CAD build for the part. Positions are in the model's coordinates, mm. Face numbers are marked on the shaded views. Round coordinates to 2 decimals unless told otherwise and drop trailing zeros. Order: outer loops, then holes, each group sorted by start corner. A loop starts at its lowest first (then second) coordinate and runs counter-clockwise, first axis right, second up. Notation, with made-up numbers: (-24.75, 55.25) - (-15.75, 55.25) arc R4 cw to (-15.75, 62.25) - close; hole circle Ø1 at (50, -25). An arc over 180 degrees is marked (long way). Write item = value, one per line.
from build123d import *

# Parameters (mm, degrees)
F1_DEPTH = 10
F2_R     = 3
F3_R     = 5


with BuildPart() as f1:
    # F0 (on Top) → F1 (new body)
    with BuildSketch(Plane.XY):
        Polygon((-6, 105.431184), (0, 105.431184), (6, 105.431184), (6, -54.568816), (4, -89.978623), (4, -107.107288), (12, -68.312444), (12, 113.431184), (0, 113.431184), (-12, 113.431184), (-12, -68.312444), (-4, -107.107288), (-4, -89.978623), (-6, -54.568816), align=None)
    extrude(amount=F1_DEPTH)

    # F2
    f2_edges = [f1.edges().sort_by_distance(p)[0] for p in [
        (6, 105.431184, 5),
        (-6, 105.431184, 5),
    ]]
    fillet(f2_edges, radius=F2_R)

    # F3
    f3_edges = [f1.edges().sort_by_distance(p)[0] for p in [
        (-12, 113.431184, 5),
        (12, 113.431184, 5),
    ]]
    fillet(f3_edges, radius=F3_R)


solid = f1.part
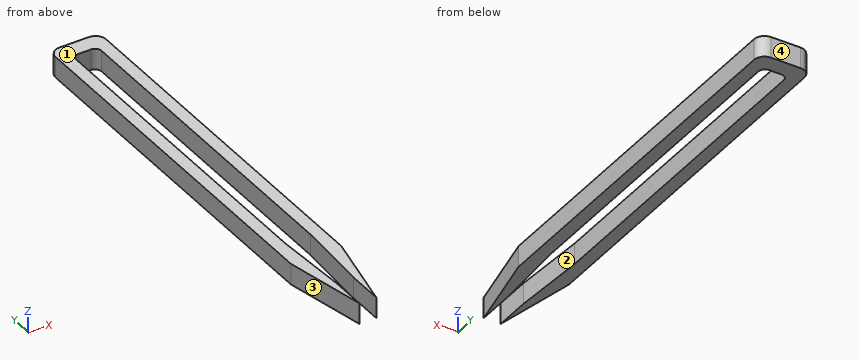
(1) Band-saw the part on C-C on x = 0. List the corners of the cut face in (y, z), plus the area to 3 significant figures.
Solved:
outline = (105.43, 0) - (113.43, 0) - (113.43, 10) - (105.43, 10) - close
area = 80.0 mm²
(2) Band-saw the part on B-B on z = 8.25. List the corners of the cut face in (x, y).
Solved:
outline = (-12, -68.31) - (-4, -107.11) - (-4, -89.98) - (-6, -54.57) - (-6, 102.43) arc R3 cw to (-3, 105.43) - (3, 105.43) arc R3 cw to (6, 102.43) - (6, -54.57) - (4, -89.98) - (4, -107.11) - (12, -68.31) - (12, 108.43) arc R5 ccw to (7, 113.43) - (-7, 113.43) arc R5 ccw to (-12, 108.43) - close
(3) Probe line 1 along X through (y, z) = (44, 0.75); line 2 along Y through (x, z) = (3.5, 3.25); line 3 along X through (y, z) = (-68, 3.75). List the from-to ranges inside material, lowest first.
Solved:
line_1 = -12 to -6, 6 to 12
line_2 = 105.39 to 113.43
line_3 = -12 to -5.24, 5.24 to 12
(4) Drop flat-ended pins along their axis: pin 1 (5 mm diameter, centred on y = -95, z = 3.5, fed in from -X); pin 2 (1.8 mm diameter, centred on x = 1.5, z = 6, fed in from -Y); pin 3 (1.5 mm diameter, centred on y = -79, z = 2, fed in from +X). Give the stop position or say it passes through.
Solved:
pin_1 = -7.01
pin_2 = 105.43
pin_3 = 9.95
(5) Band-saw the part on A-A on y = 70. List the corners of the cut face in (x, z).
Solved:
outline = (-12, 0) - (-6, 0) - (-6, 10) - (-12, 10) - close; (6, 0) - (12, 0) - (12, 10) - (6, 10) - close
(6) Pull direction Y, two halves, no side cores. Call the marked faces 1, 2, 3 and 4: released by +Y, released by -Y, zero draft, split by the parting line, or undercut.
Solved:
face_1 = zero draft
face_2 = undercut
face_3 = released by -Y
face_4 = released by +Y
(7) Band-saw the part on D-D on y = -79. List the corners of the cut face in (x, z), plus the area to 3 significant figures.
Solved:
outline = (-9.8, 0) - (-4.62, 0) - (-4.62, 10) - (-9.8, 10) - close; (4.62, 0) - (9.8, 0) - (9.8, 10) - (4.62, 10) - close
area = 104 mm²
